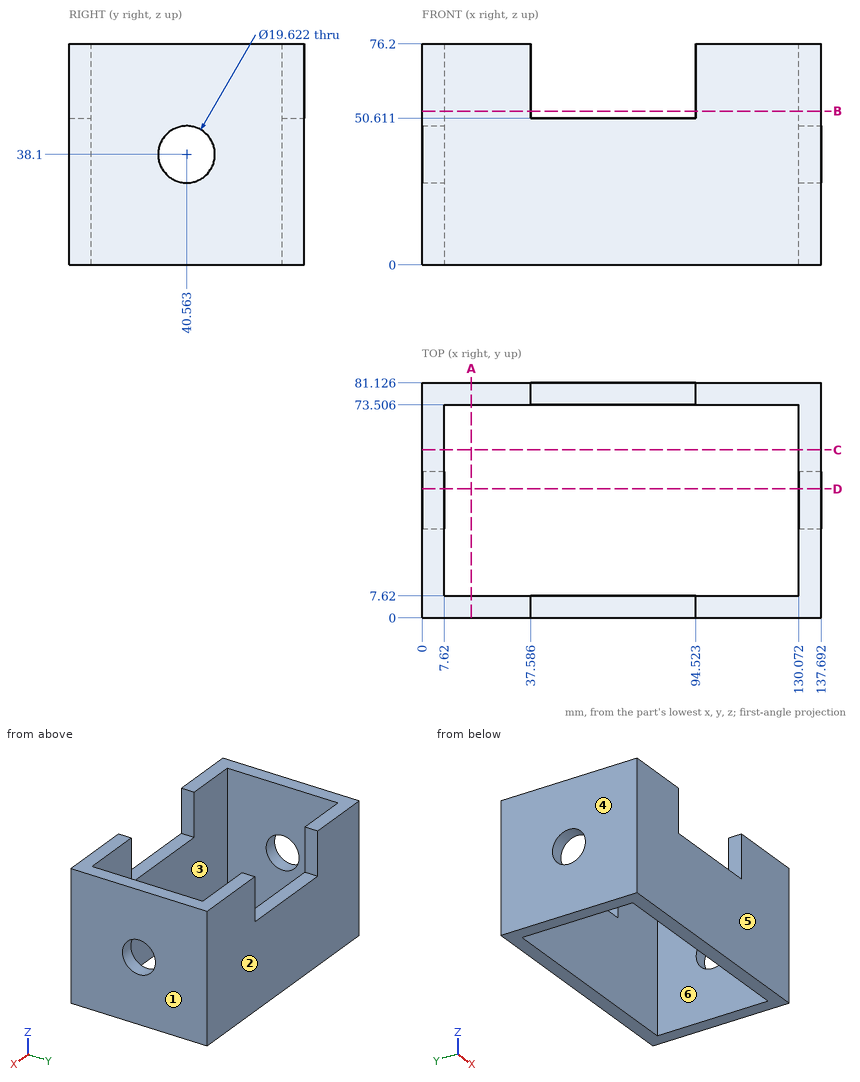
Verification items for this drawing (mm, ordinates from the low corner). A direction names the side the tool comes from. Round coordinates to 2 decimals unless told otherwise and drop trailing zeros. Write each loop counter-clockwise with the first axis right and the second up, starting at its lowest first coordinate (ties: lowest second). Pieces come first, ordered by that corner, then holes. Notation, with made-up numbers: (87, 8.25) - (99, 8.25) arc R34 ccw to (99, 47.25) - close; hole circle Ø2 at (77.25, 53.5). An arc over 180 degrees is marked (long way). One line per item, written item: value.
1. Cross-section at C-C on y = 58. Record the boundary of the cut face in (x, z), and give its area (3 significant figures).
The answers:
outline: (0, 0) - (7.62, 0) - (7.62, 76.2) - (0, 76.2) - close; (130.07, 0) - (137.69, 0) - (137.69, 76.2) - (130.07, 76.2) - close
area: 1,160 mm^2
2. Cross-section at A-A on x = 17. Record the boundary of the cut face in (y, z).
The answers:
outline: (0, 0) - (7.62, 0) - (7.62, 76.2) - (0, 76.2) - close; (73.51, 0) - (81.13, 0) - (81.13, 76.2) - (73.51, 76.2) - close
3. Cross-section at D-D on y = 44.5. Record the boundary of the cut face in (x, z).
The answers:
outline: (0, 0) - (7.62, 0) - (7.62, 29.11) - (0, 29.11) - close; (0, 47.09) - (7.62, 47.09) - (7.62, 76.2) - (0, 76.2) - close; (130.07, 0) - (137.69, 0) - (137.69, 29.11) - (130.07, 29.11) - close; (130.07, 47.09) - (137.69, 47.09) - (137.69, 76.2) - (130.07, 76.2) - close
4. Scan lines: L1, parallel to Y at x = 116, z = 40.5; L2, parallel to X at y = 52, z = 43. Record each from-to range of solid material in increasing order.
The answers:
L1: y = 0 to 7.62, 73.51 to 81.13
L2: x = 0 to 7.62, 130.07 to 137.69
5. Mould release check, pull along X, two halves, no side actions. Record for the marked faces 1, 2, 3 and 4: released by +X, released by -X, zero draft, split by the parting line, or undercut.
The answers:
face 1: released by +X
face 2: zero draft
face 3: undercut
face 4: released by -X
6. Cross-section at B-B on z = 53. Record the boundary of the cut face in (x, y).
The answers:
outline: (0, 0) - (37.59, 0) - (37.59, 7.62) - (7.62, 7.62) - (7.62, 73.51) - (37.59, 73.51) - (37.59, 81.13) - (0, 81.13) - close; (94.52, 0) - (137.69, 0) - (137.69, 81.13) - (94.52, 81.13) - (94.52, 73.51) - (130.07, 73.51) - (130.07, 7.62) - (94.52, 7.62) - close
7. Set-up check for the marked faces 5 and 6: record each of +Z, -Z, +X, -X, +Y, -Y from which the full face is reachable in a straight line by a thin tool's end or side.
The answers:
face 5: +Z, -Z, +X, -X, -Y
face 6: +Z, -Z
8. Depth check by flat-ended pin: pin 1 Ø4 at (x, y) = (54, 3.5) entering from +Z. Enter the tip coordinate at first touch or a pass-through.
The answers:
pin 1: stops at z = 50.61
